Design review of the part shown in the three views and the two pictorial views. Dimensions are in mm from the part's minimum x, y and z. A direction names the side the tool comes from. Round coordinates to 2 decimals unless told otherwise and drop trailing zeros. Loops run counter-clockwise (first coordinate to the right, second up) from the corner with the lowest first, then second, coordinate; pieces in that order, holes last.
1. Draft analysis for pull direction Z (two halves, no side actions). For the marked faces 1 and 2, state which applies: released by +Z, released by -Z, zero draft, split by the parting line, or undercut.
2. To check wall thickness, follow line 1 along Z through (x, y) = (17.7, 16.1); line 2 along Y through (x, z) = (6, 35); line 3 along Y through (x, z) = (10.25, 12). State the ranges of each line that lie inside material, in increasing order.
3. Consider section D-D on y = 6.5. State the section outline as (x, z) points.
4. Clearance check with flat-ended pins moving along their axes: pin 1 Ø3.5 at (x, z) = (2.3, 12.3) entering from +Y; pin 2 Ø1.1 at (x, y) = (11.5, 13.5) entering from -Z; pin 3 Ø5 at (y, z) = (13.5, 5) entering from +X. State where each tip first meets the part, or that it passes through.
5. Consider section A-A on x = 1.5. State the section outline as (y, z) points.
6. Consider section C-C on x = 10. State the section outline as (y, z) points.
7. Consider section B-B on z = 36. State the section outline as (x, y) points.
8. Tool access review of the marked faces 3, 4, 5, 6 and 7: name each direction out of +Z, -Z, +X, -X, +Y, -Y from which nothing blocks a thin tool from reaching the whole face with its end or side.
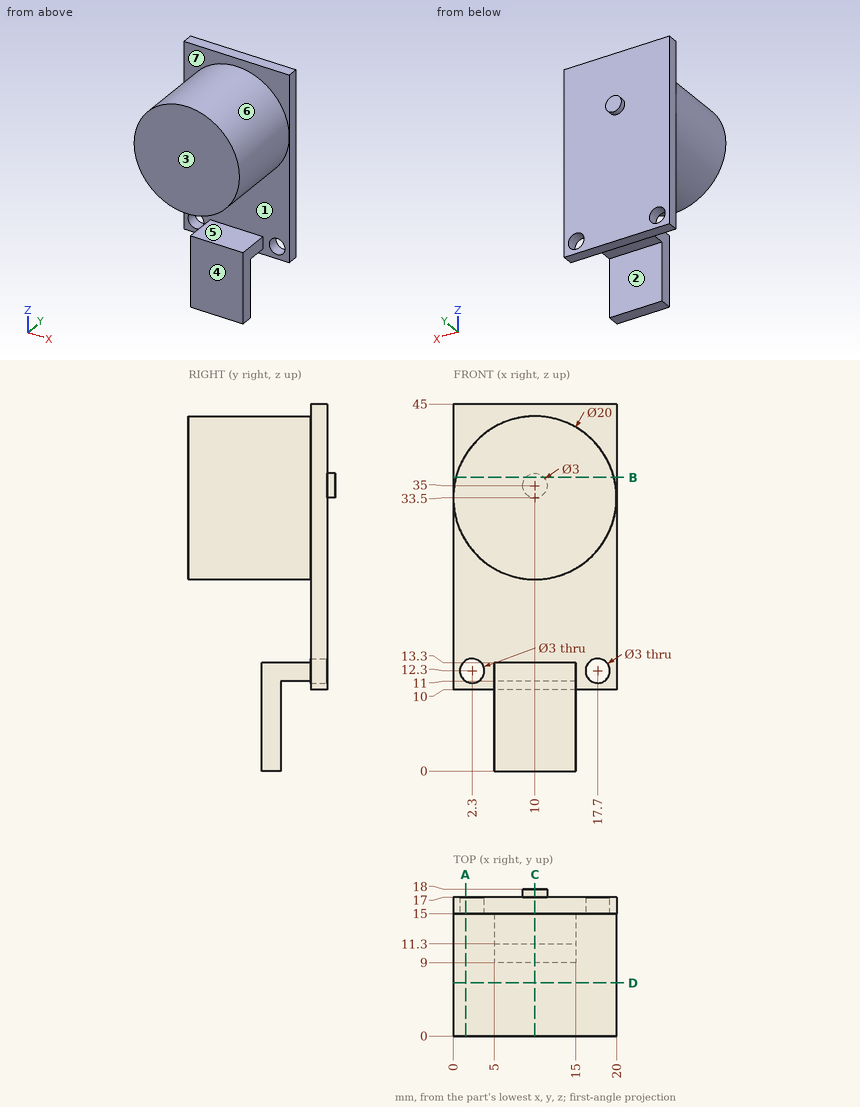
Resolved:
1. face 1: undercut
1. face 2: zero draft
2. line 1: z = 10 to 10.8, 13.8 to 45
2. line 2: y = 0 to 17
2. line 3: y = 9 to 17
3. outline: circle Ø20 at (10, 33.5)
4. pin 1: stops at y = 17
4. pin 2: stops at z = 11
4. pin 3: stops at x = 15
5. outline: (0, 28.23) - (15, 28.23) - (15, 13.57) - (17, 13.57) - (17, 45) - (15, 45) - (15, 38.77) - (0, 38.77) - close; (15, 10) - (17, 10) - (17, 11.03) - (15, 11.03) - close
6. outline: (0, 23.5) - (15, 23.5) - (15, 13.3) - (9, 13.3) - (9, 0) - (11.3, 0) - (11.3, 11) - (15, 11) - (15, 10) - (17, 10) - (17, 33.5) - (18, 33.5) - (18, 36.5) - (17, 36.5) - (17, 45) - (15, 45) - (15, 43.5) - (0, 43.5) - close
7. outline: (0, 15) - (0.32, 15) - (0.32, 0) - (19.68, 0) - (19.68, 15) - (20, 15) - (20, 17) - (11.12, 17) - (11.12, 18) - (8.88, 18) - (8.88, 17) - (0, 17) - close
8. face 3: +Z, -Z, +X, -X, -Y
8. face 4: -Z, +X, -X, -Y
8. face 5: +X, -X, -Y
8. face 6: -Y
8. face 7: +Z, -Y
